Model file for the job. Use its own axes, mm. Round coordinates to 2 decimals unless told otherwise and drop trailing zeros. Loops run counter-clockwise (first coordinate to the right, second up) from the corner with the lowest first, then second, coordinate; pieces in that order, holes last. Notation, with made-up numbers: M 1.5,81.5 L 5.5,81.5 A34 cw 5.5,114.5 Z; hole C 59.25,19.5 d11. An arc over 180 degrees is marked long. Use a Markdown table: item, result. Add a question column.
Item 1: Saw through at D-D on z = 44. Write the cut outline in (x, y).
Item 2: Saw through at A-A on z = 22. Write the cut outline in (x, y).
Item 3: Pin check, flat tips, straight feed: P1, Ø8, axis at y = 6, z = 4, coming from the -X side; P2, Ø2.5, axis at y = 6, z = 62, coming from the +X side. Stop position of each tip, or through.
Item 4: Wall check: L1, parallel to Z at x = -0.85, y = -6; L2, parallel to Y at x = 0.45, z = 43; L3, parallel to Y at x = 1.1, z = 4. Give the ranges that are in metal, low to high. Write a range as from..to.
Item 5: Saw through at B-B on x = 0.2. Give the number of separate pieces and of enclosed holes in the cut face, then the cut area to 3 significant figures.
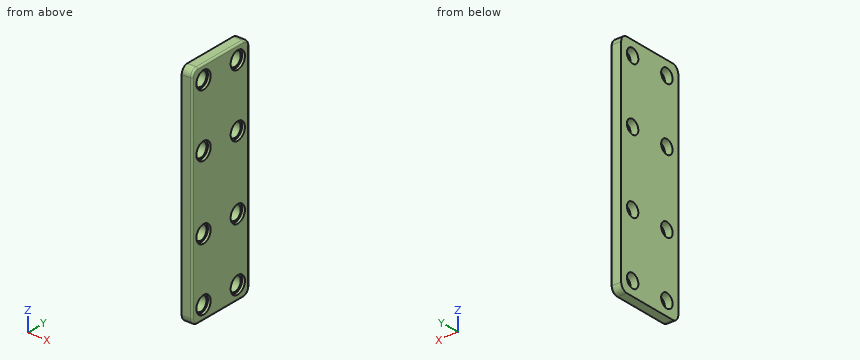
```python
from build123d import *

# Parameters (mm, degrees)
SKETCH2_W            = 3
SKETCH2_H            = 20
BOSS_EXTRUDE2_DEPTH  = 65
FILLET3_R            = 2
FILLET4_R            = 2
FILLET5_R            = 2
FILLET6_R            = 2
LPATTERN1_COUNT      = 2
LPATTERN1_PITCH      = 18
LPATTERN1_COUNT_DIR2 = 2
LPATTERN1_PITCH_DIR2 = 12
FILLET7_R            = 0.5


with BuildPart() as part:
    # Sketch2 → Boss-Extrude2 (new body)
    with BuildSketch(Plane.XY):
        Rectangle(SKETCH2_W, SKETCH2_H)
    extrude(amount=BOSS_EXTRUDE2_DEPTH)

    # Fillet3
    fillet3_edges = [part.edges().sort_by_distance(p)[0] for p in [
        (0, 10, 65),
    ]]
    fillet(fillet3_edges, radius=FILLET3_R)

    # Fillet4
    fillet4_edges = [part.edges().sort_by_distance(p)[0] for p in [
        (0, -10, 65),
    ]]
    fillet(fillet4_edges, radius=FILLET4_R)

    # Fillet5
    fillet5_edges = [part.edges().sort_by_distance(p)[0] for p in [
        (0, 10, 0),
    ]]
    fillet(fillet5_edges, radius=FILLET5_R)

    # Fillet6
    fillet6_edges = [part.edges().sort_by_distance(p)[0] for p in [
        (0, -10, 0),
    ]]
    fillet(fillet6_edges, radius=FILLET6_R)

    # Sketch4 → CBORE for M5 Hex Head Bolt1 (revolve, cut)
    with BuildSketch(Plane(origin=(1.5, 6, 61), x_dir=(0, 0, -1), z_dir=(0, 1, 0))):
        Polygon((0, 0), (0, 5.178090033), (2, 4), (2, 0.8), (2.5, 0.8), (2.5, 0), align=None)
    cbore_for_m5_hex_head_bolt1 = revolve(axis=Axis((7.85, 6, 61), (-1, 0, 0)), mode=Mode.SUBTRACT)

    # LPattern1: CBORE for M5 Hex Head Bolt1 2 × 2
    with Locations(*[(0, -j * LPATTERN1_PITCH_DIR2, -i * LPATTERN1_PITCH) for i in range(LPATTERN1_COUNT) for j in range(LPATTERN1_COUNT_DIR2) if (i, j) != (0, 0)]):
        add(cbore_for_m5_hex_head_bolt1, mode=Mode.SUBTRACT)

    # Mirror16: CBORE for M5 Hex Head Bolt1 across plane
    add(cbore_for_m5_hex_head_bolt1.mirror(Plane.XY.offset(32.5)), mode=Mode.SUBTRACT)

    # Mirror16 copy 1 sketch → Mirror16 copy 1 (revolve, cut)
    with BuildSketch(Plane(origin=(1.5, -6, 4), x_dir=(0, 0, 1), z_dir=(0, 1, 0))):
        Polygon((0, 0), (0, -5.178090033), (2, -4), (2, -0.8), (2.5, -0.8), (2.5, 0), align=None)
    revolve(axis=Axis((7.85, -6, 4), (1, 0, 0)), mode=Mode.SUBTRACT)

    # Mirror16 copy 2 sketch → Mirror16 copy 2 (revolve, cut)
    with BuildSketch(Plane(origin=(1.5, 6, 22), x_dir=(0, 0, 1), z_dir=(0, 1, 0))):
        Polygon((0, 0), (0, -5.178090033), (2, -4), (2, -0.8), (2.5, -0.8), (2.5, 0), align=None)
    revolve(axis=Axis((7.85, 6, 22), (1, 0, 0)), mode=Mode.SUBTRACT)

    # Mirror16 copy 3 sketch → Mirror16 copy 3 (revolve, cut)
    with BuildSketch(Plane(origin=(1.5, -6, 22), x_dir=(0, 0, 1), z_dir=(0, 1, 0))):
        Polygon((0, 0), (0, -5.178090033), (2, -4), (2, -0.8), (2.5, -0.8), (2.5, 0), align=None)
    revolve(axis=Axis((7.85, -6, 22), (1, 0, 0)), mode=Mode.SUBTRACT)

    # Fillet7
    fillet7_edges = [part.edges().sort_by_distance(p)[0] for p in [
        (1.5, 10, 32.5),
        (1.5, 9.414213562, 64.414213562),
        (1.5, 0, 65),
        (1.5, -10, 32.5),
        (1.5, -9.414213562, 64.414213562),
        (1.5, 9.414213562, 0.585786438),
        (1.5, 0, 0),
        (1.5, -9.414213562, 0.585786438),
    ]]
    fillet(fillet7_edges, radius=FILLET7_R)


solid = part.part
```
Entries:
| question | item | result |
|---|---|---|
| 1 | outline | M -1.5,-10 L 1,-10 A0.5 ccw 1.5,-9.5 L 1.5,-8.29 L 0.7,-8.29 L 0.7,-7.73 L -1.5,-7.73 Z; M -1.5,-4.27 L 0.7,-4.27 L 0.7,-3.71 L 1.5,-3.71 L 1.5,3.71 L 0.7,3.71 L 0.7,4.27 L -1.5,4.27 Z; M -1.5,7.73 L 0.7,7.73 L 0.7,8.29 L 1.5,8.29 L 1.5,9.5 A0.5 ccw 1,10 L -1.5,10 Z |
| 2 | outline | M -1.5,-10 L 1,-10 A0.5 ccw 1.5,-9.5 L 1.5,-8.5 L 0.7,-8.5 L 0.7,-8 L -1.5,-8 Z; M -1.5,-4 L 0.7,-4 L 0.7,-3.5 L 1.5,-3.5 L 1.5,3.5 L 0.7,3.5 L 0.7,4 L -1.5,4 Z; M -1.5,8 L 0.7,8 L 0.7,8.5 L 1.5,8.5 L 1.5,9.5 A0.5 ccw 1,10 L -1.5,10 Z |
| 3 | P1 | x = -1.5 |
| 3 | P2 | x = 0.7 |
| 4 | L1 | 0..2, 6..20, 24..41, 45..59, 63..65 |
| 4 | L2 | -10..-8, -4..4, 8..10 |
| 4 | L3 | -9.99..-8.5, -3.5..3.5, 8.5..9.99 |
| 5 | separate pieces | 1 |
| 5 | enclosed holes | 8 |
| 5 | area | 1,200 mm2 |
